Here's how the part is built. I have some questions about the finished solid (model axes, mm). A direction names the side the tool comes from. Give positions to 0.01 mm unless a question says otherwise; leave off trailing zeros. Write each loop counter-clockwise with the first axis right and the second up, starting at its lowest first coordinate (ties: lowest second). Pieces come first, ordered by that corner, then holes. Notation, with made-up numbers: M 25.5,58 L 77.5,58 A12 ccw 77.5,63 Z; hole C 35,-3.5 d4. An arc over 180 degrees is marked long. Use one line per item in the form item = value. Start each with the question number.
from build123d import *

# Parameters (mm, degrees)
F0_R     = 15
F0_R_2   = 10
F1_DEPTH = 20
F2_R     = 37.5
F2_R_2   = 15
F2_R_3   = 10
F3_DEPTH = 10
F4_R     = 25
F4_R_2   = 10
F5_DEPTH = 30
F6_R     = 37.5
F6_R_2   = 25
F6_R_3   = 10
F7_DEPTH = 10


with BuildPart() as f1:
    # F0 (on Right) → F1 (new body)
    with BuildSketch(Plane.YZ):
        Circle(F0_R)
        Circle(F0_R_2, mode=Mode.SUBTRACT)
    extrude(amount=F1_DEPTH)

    # F2 (on face) → F3 (join)
    with BuildSketch(Plane.YZ.offset(20)):
        Circle(F2_R)
        Circle(F2_R_2, mode=Mode.SUBTRACT)
        Circle(F2_R_2)
        Circle(F2_R_3, mode=Mode.SUBTRACT)
    extrude(amount=F3_DEPTH)

    # F4 (on face) → F5 (join)
    with BuildSketch(Plane.YZ.offset(30)):
        Circle(F4_R)
        Circle(F4_R_2, mode=Mode.SUBTRACT)
    extrude(amount=F5_DEPTH)

    # F6 (on face) → F7 (join)
    with BuildSketch(Plane.YZ.offset(60)):
        Circle(F6_R)
        Circle(F6_R_2, mode=Mode.SUBTRACT)
        Circle(F6_R_2)
        Circle(F6_R_3, mode=Mode.SUBTRACT)
    extrude(amount=F7_DEPTH)


solid = f1.part
1) Will these pins go through, and if not, where does the flat tip stop? P1, Ø3, axis at x = 50, y = -8.5, coming from the -Z side; P2, Ø6, axis at x = 56, y = 3.5, coming from the -Z side (3 decimals); P3, Ø10, axis at x = 27.5, y = 0.5, coming from the -Z side.
2) Suppose I cut it at C-C, the plane x = 65.5. List the corners of the cut face in (y, z) for me.
3) Thinking about a two-plate mould opening in Y: for faces 4 (the face through (34.51, -2.17, -9.76)), 5 (the face through (60, 24, -8)), 6 (the face through (24.93, -4.88, 37.18)), which applies, released by +Y, released by -Y, zero draft, split by the parting line, or undercut?
4) On a 3-axis mill with a long thin cutter (end or side, diameter ignored), from which of +Z, -Z, +X, -X, +Y, -Y can I reach the whole of each face in a straight line? I mean faces 1 (the face through (44.79, 23.846, 7.509)), 2 (the face through (20, 16, 1)), 3 (the face through (64.93, -4.88, 37.18)). Say none if no direction works.
5) Suppose I cut it at D-D, the plane y = -20.5. List the corners of the cut face in (x, z) for me.
6) Please list where these lines run through material, in increasing order: line 1 (X direction, y = -26, z = -21.5); line 2 (Z direction, x = 44.5, y = 0); line 3 (Z direction, x = 28, y = 0).
7) Suppose I cut it at A-A, the plane z = 0. List the corners of the cut face in (x, y) for me, and give its area (3 significant figures).
Checks:
q1.P1 = -24
q1.P2 = -24.995
q1.P3 = -37.5
q2.outline = C 0,0 d75; hole C 0,0 d20
q3.face_4 = undercut
q3.face_5 = zero draft
q3.face_6 = split by the parting line
q4.face_1 = none
q4.face_2 = -X
q4.face_3 = +X, -X
q5.outline = M 20,-31.4 L 30,-31.4 L 30,-14.31 L 60,-14.31 L 60,-31.4 L 70,-31.4 L 70,31.4 L 60,31.4 L 60,14.31 L 30,14.31 L 30,31.4 L 20,31.4 Z
q6.line_1 = 20 to 30, 60 to 70
q6.line_2 = -25 to -10, 10 to 25
q6.line_3 = -37.5 to -10, 10 to 37.5
q7.outline = M 0,-15 L 20,-15 L 20,-37.5 L 30,-37.5 L 30,-25 L 60,-25 L 60,-37.5 L 70,-37.5 L 70,-10 L 0,-10 Z; M 0,10 L 70,10 L 70,37.5 L 60,37.5 L 60,25 L 30,25 L 30,37.5 L 20,37.5 L 20,15 L 0,15 Z
q7.area = 2,200 mm^2
